Source: CAD feature listing. Evaluate the final solid. Frame: model axes, mm. A direction names the side the tool comes from. Coordinates: 2 decimals unless noted, no trailing zeros. Write each loop counter-clockwise with the first axis right and the second up, starting at its lowest first coordinate (ties: lowest second). Pieces come first, ordered by that corner, then holes. Notation, with made-up numbers: (85.25, 70) - (98.25, 70) arc R21 ccw to (98.25, 96) - close; hole circle Ø9 at (14, -35.75). An arc over 180 degrees is marked (long way). One line per item, written item: value.
from build123d import *

# Parameters (mm, degrees)
FILLET1_R    = 1
RECPAT_COUNT = 2
RECPAT_ANGLE = 90


with BuildPart() as part:
    # BodySke → Base-Revolve (revolve)
    with BuildSketch(Plane.XY, mode=Mode.PRIVATE) as base_revolve_sk:
        Polygon((0, 0), (0, 4.2), (0.5, 4.2), (2.7, 2), (20, 2), (20, 0), align=None)
    revolve(base_revolve_sk.sketch.rotate(Axis((-6.35, 0, 0), (1, 0, 0)), 90), axis=Axis((-6.35, 0, 0), (1, 0, 0)))

    # Fillet1
    fillet1_edges = [part.edges().sort_by_distance(p)[0] for p in [
        (2.7, 0, -2),
    ]]
    fillet(fillet1_edges, radius=FILLET1_R)

    # Sketch3 → Recess section 0
    with BuildSketch(Plane.ZY):
        with BuildLine():
            Line((-0.515, 2.2), (0.515, 2.2))
            Line((0.515, 2.2), (0.515, -2.2))
            Line((0.515, -2.2), (-0.515, -2.2))
            Line((-0.515, -2.2), (-0.515, 2.2))
        make_face()
    # Sketch4 → Recess section 1
    with BuildSketch(Plane.ZY.offset(-2.51)):
        with BuildLine():
            Line((-0.515, 0.948560207), (0.515, 0.948560207))
            Line((0.515, 0.948560207), (0.515, -0.948560207))
            Line((0.515, -0.948560207), (-0.515, -0.948560207))
            Line((-0.515, -0.948560207), (-0.515, 0.948560207))
        make_face()
    recess = loft(mode=Mode.SUBTRACT)

    # RecPat: Recess ×2 about axis
    recpat_axis = Axis((0, 0, 0), (1, 0, 0))
    for i in range(1, RECPAT_COUNT):
        add(recess.rotate(recpat_axis, i * RECPAT_ANGLE / (RECPAT_COUNT - 1)), mode=Mode.SUBTRACT)

    # RecCorSke → RecessCore (revolve, cut)
    with BuildSketch(Plane.XY, mode=Mode.PRIVATE) as recesscore_sk:
        Polygon((0, 0), (0, 1.026516298), (2.51, 0.851), (2.786506661, 0), align=None)
    revolve(recesscore_sk.sketch.rotate(Axis((-3.175, 0, 0), (1, 0, 0)), 90), axis=Axis((-3.175, 0, 0), (1, 0, 0)), mode=Mode.SUBTRACT)


solid = part.part
1) Section query A-A on x = 14. Output: boundary loops of the cut face in (y, z).
Values found:
outline: circle Ø4 at (0, 0)
2) Draft query along Y for faces 1 (the flat face through (20, 0, 0)), 2 (the cylindrical face through (0.254, -1.262, 4.006)), 3 (the conical face through (2.77, 0.04, 0.02)). Return one class per face: released by +Y, released by -Y, zero draft, split by the parting line, or undercut.
Values found:
face 1: zero draft
face 2: split by the parting line
face 3: undercut
3) Contact query for flat-ended pins moving along their axis: P1, Ø2, axis at x = 4.5, z = 0, coming from the +Y side; P2, Ø1, axis at x = 14, y = -1, coming from the +Z side; P3, Ø4, axis at x = 15.5, y = -1, coming from the -Z side. Output: stop coordinate, or through.
Values found:
P1: y = 2
P2: z = 1.94
P3: z = -2
4) Material intervals for line 1 (Z direction, x = 1.5, y = 0.75); line 2 (Y direction, x = 2.25, z = -1) (3 decimals); line 3 (X direction, y = 2, z = 1.5), sorted ascending.
Values found:
line 1: -3.11 to -0.54, 0.54 to 3.11
line 2: -2.237 to -0.515, 0.515 to 2.237
line 3: 0 to 2.2
5) Reachability of faces 4 (the flat face through (0, 1, -1)), 5 (the cylindrical face through (12, 2, 0)), 6 (the flat face through (1.273, -1.566, 0.007)) from +Z, -Z, +X, -X, +Y, -Y: full face, straight path, thin tool, end or side. Return the list, or none.
Values found:
face 4: +Z, -Z, -X, +Y, -Y
face 5: +X
face 6: -X
